For this review, use the dimensioned drawing (mm, ordinates from the lowest corner) and the shaded views. A direction names the side the tool comes from. Give positions to 0.01 mm unless a question says otherwise; leave off trailing zeros. Order: outer loops, then holes, each group sorted by start corner. A loop starts at its lowest first (then second) coordinate and runs counter-clockwise, first axis right, second up. Notation, with made-up numbers: M -17,62.25 L -2,62.25 A19 cw -2,72.25 Z; hole C 38.5,-38 d8. An arc over 180 degrees is marked long. One line per question, with ' | ' between items. Start each with the question number.
1. The part is to be moulded in two halves that separate along X. For the marked faces 1, 2 and 3, say which applies: +X half, -X half, draft (parallel to the pull), parting line (faces both ways), or undercut.
2. Insertion check: P1, Ø22, axis at x = 36.5, y = 46.5, coming from the +Z side. The pin has a flat end and moves straight along its axis. Give the tip position at first contact, or say it passes through.
3. For the marked faces 4 and 5, list the 3-axis set-ups (+Z, -Z, +X, -X, +Y, -Y) from which the entire face can be reached by the end or side of a thin tool; tool diameter is ignored.
4. We need section C-C on x = 27. Write out the cut boundary in (y, z).
5. We need section B-B on z = 21.5. Write out the cut boundary in (x, y), then the cut area to 3 significant figures.
6. We need section A-A on y = 57.5. Write out the cut boundary in (x, z).
7. Wall thickness on L1, parallel to X at y = 14, z = 15; L2, parallel to Z at x = 48.5, y = 32; L3, parallel to X at y = 8.5, z = 2 (1 decimal): over which ranges is each line inside the solid? List them lowest first.
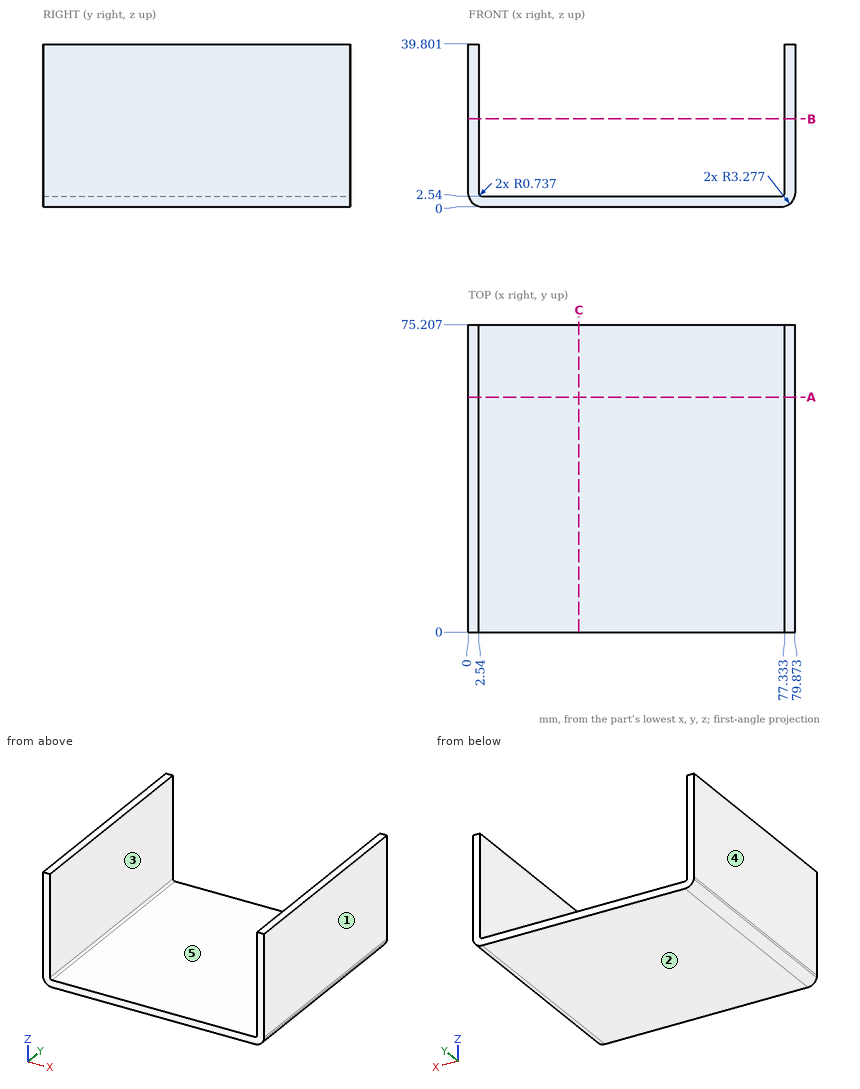
Entries:
1) face 1: +X half | face 2: draft | face 3: undercut
2) P1: stops at z = 2.54
3) face 4: +Z, -Z, -X, +Y, -Y | face 5: +Z, +Y, -Y
4) outline: M 0,0 L 75.21,0 L 75.21,2.54 L 0,2.54 Z
5) outline: M 0,0 L 2.54,0 L 2.54,75.21 L 0,75.21 Z; M 77.33,0 L 79.87,0 L 79.87,75.21 L 77.33,75.21 Z | area: 382 mm^2
6) outline: M 0,3.28 A3.28 ccw 3.28,0 L 76.6,0 A3.28 ccw 79.87,3.28 L 79.87,39.8 L 77.33,39.8 L 77.33,3.28 A0.74 cw 76.6,2.54 L 3.28,2.54 A0.74 cw 2.54,3.28 L 2.54,39.8 L 0,39.8 Z
7) L1: x = 0 to 2.54, 77.33 to 79.87 | L2: z = 0 to 2.54 | L3: x = 0.3 to 79.6
